Can you work these out from the model? Positions are in its coordinate system, mm. A direction names the side the tool comes from. Round coordinates to 2 decimals unless told otherwise and drop trailing zeros. Write each loop counter-clockwise with the first axis right and the second up, starting at its lowest first coordinate (ties: lowest second). Pieces come first, ordered by that corner, then holes. Notation, with made-up numbers: (83.5, 32.5) -> (101.5, 32.5) arc R17 cw to (101.5, 56.5) -> close; hole circle Ø11 at (6, -7). An arc over 180 degrees is marked (long way). Use CSV: the item, a comma, the result in double quotes.
```python
from build123d import *

# Parameters (mm, degrees)
SKETCH_1_W                   = 46
SKETCH_1_H                   = 26
EXTRUDE_1_DEPTH              = 5
SKETCH_2_W                   = 3
SKETCH_2_H                   = 26
EXTRUDE_2_DEPTH              = 34
FILLET_1_R                   = 13
CUT_EXTRUDE_1_REACH          = 63.693
SKETCH_3_R                   = 4
HOLE_WIZARD_M2_1_D           = 2.4
HOLE_WIZARD_M2_1_CBORE_D     = 4.4
HOLE_WIZARD_M2_1_CBORE_DEPTH = 2
SKETCH_6_W                   = 39
SKETCH_6_H                   = 25
CUT_EXTRUDE_3_DEPTH          = 3
CHAMFER_1_SIZE               = 3
SKETCH_7_W                   = 8
SKETCH_7_H                   = 5
CUT_EXTRUDE_4_DEPTH          = 10
SKETCH_8_W                   = 5
SKETCH_8_H                   = 5
CUT_EXTRUDE_5_DEPTH          = 10
SKETCH_9_R                   = 2.7
EXTRUDE_7_DEPTH              = 1
HOLE_WIZARD_M2_2_D           = 2.4
HOLE_WIZARD_M2_2_CBORE_D     = 4.4
HOLE_WIZARD_M2_2_CBORE_DEPTH = 2
M2X0_4_1_D                   = 1.6


with BuildPart() as part:
    # 草图1 → 凸台-拉伸1 (new body)
    with BuildSketch(Plane(origin=(0, 0, 0), x_dir=(1, 0, 0), z_dir=(0, 1, 0))):
        Rectangle(SKETCH_1_W, SKETCH_1_H)
    extrude(amount=EXTRUDE_1_DEPTH)

    # 草图2 → 凸台-拉伸2 (add)
    with BuildSketch(Plane(origin=(0, 5, 0), x_dir=(1, 0, 0), z_dir=(0, 1, 0))):
        with Locations((-21.5, 0)):
            Rectangle(SKETCH_2_W, SKETCH_2_H)
        with Locations((21.5, 0)):
            Rectangle(SKETCH_2_W, SKETCH_2_H)
    extrude(amount=EXTRUDE_2_DEPTH)

    # 圆角1
    fillet_1_edges = [part.edges().sort_by_distance(p)[0] for p in [
        (21.5, 39, -13),
        (-21.5, 39, -13),
        (21.5, 39, 13),
        (-21.5, 39, 13),
    ]]
    fillet(fillet_1_edges, radius=FILLET_1_R - 0.0001)  # a hair under: the kernel refuses the full size

    # 草图3 → 切除-拉伸1 (cut, up to next)
    with BuildSketch(Plane.ZY.offset(23), mode=Mode.PRIVATE) as cut_extrude_1_sk1:
        with Locations((0, 26)):
            Circle(SKETCH_3_R)
    cut_extrude_1_tool1 = extrude(cut_extrude_1_sk1.sketch, amount=-CUT_EXTRUDE_1_REACH, mode=Mode.PRIVATE) & part.part
    cut_extrude_1 = cut_extrude_1_tool1.solids().sort_by_distance((-23, 26, 0))[0]
    add(cut_extrude_1, mode=Mode.SUBTRACT)

    # M2 凹头盖螺钉的柱形沉头孔1 (through all)
    with Locations(Plane(origin=(-23, 26, -8), x_dir=(0, 0, -1), z_dir=(-1, 0, 0))):
        with Locations((0, 0), (-8, -8), (-16, 0), (-8, 8)):
            hole_wizard_m2_1 = CounterBoreHole(HOLE_WIZARD_M2_1_D / 2, HOLE_WIZARD_M2_1_CBORE_D / 2, HOLE_WIZARD_M2_1_CBORE_DEPTH)

    # 镜向1: 切除-拉伸1, M2 凹头盖螺钉的柱形沉头孔1 across plane
    add(cut_extrude_1.mirror(Plane(origin=(0, 0, 0), x_dir=(0, 0, 1), z_dir=(1, 0, 0))), mode=Mode.SUBTRACT)
    add(hole_wizard_m2_1.mirror(Plane(origin=(0, 0, 0), x_dir=(0, 0, 1), z_dir=(1, 0, 0))), mode=Mode.SUBTRACT)

    # 草图6 → 切除-拉伸3 (cut)
    with BuildSketch(Plane(origin=(0, 5, 0), x_dir=(1, 0, 0), z_dir=(0, 1, 0))):
        Rectangle(SKETCH_6_W, SKETCH_6_H)
    extrude(amount=-CUT_EXTRUDE_3_DEPTH, mode=Mode.SUBTRACT)

    # 倒角1
    chamfer_1_edges = [part.edges().sort_by_distance(p)[0] for p in [
        (-23, 0, 0),
        (23, 0, 0),
    ]]
    chamfer(chamfer_1_edges, length=CHAMFER_1_SIZE)

    # 草图7 → 切除-拉伸4 (cut)
    with BuildSketch(Plane(origin=(23, 0, 0), x_dir=(0, 0, -1), z_dir=(1, 0, 0))):
        with Locations((0, 3.5)):
            Rectangle(SKETCH_7_W, SKETCH_7_H)
    cut_extrude_4 = extrude(amount=-CUT_EXTRUDE_4_DEPTH, mode=Mode.SUBTRACT)

    # 镜向2: 切除-拉伸4 across plane
    add(cut_extrude_4.mirror(Plane(origin=(0, 0, 0), x_dir=(0, 0, 1), z_dir=(1, 0, 0))), mode=Mode.SUBTRACT)

    # 草图8 → 切除-拉伸5 (cut)
    with BuildSketch(Plane(origin=(0, 2, 0), x_dir=(1, 0, 0), z_dir=(0, 1, 0))):
        Rectangle(SKETCH_8_W, SKETCH_8_H)
    extrude(amount=-CUT_EXTRUDE_5_DEPTH, mode=Mode.SUBTRACT)

    # 草图9 → 凸台-拉伸7 (add)
    with BuildSketch(Plane(origin=(0, 2, 0), x_dir=(1, 0, 0), z_dir=(0, 1, 0))):
        with Locations(Location((-5, 5, 0), (0, 0, 270))):
            Circle(SKETCH_9_R)
        with Locations(Location((5, 5, 0), (0, 0, 270))):
            Circle(SKETCH_9_R)
        with Locations(Location((5, -5, 0), (0, 0, 270))):
            Circle(SKETCH_9_R)
        with Locations(Location((-5, -5, 0), (0, 0, 270))):
            Circle(SKETCH_9_R)
    extrude(amount=EXTRUDE_7_DEPTH)

    # M2 凹头盖螺钉的柱形沉头孔2 (through all)
    with Locations(Plane(origin=(-5, 3, 5), x_dir=(0, 0, 1), z_dir=(0, 1, 0))):
        with Locations((0, 0), (0, 10), (-10, 10), (-10, 0)):
            CounterBoreHole(HOLE_WIZARD_M2_2_D / 2, HOLE_WIZARD_M2_2_CBORE_D / 2, HOLE_WIZARD_M2_2_CBORE_DEPTH)

    # M2x0.4 螺纹孔1 (through all)
    with Locations(Plane(origin=(-5, 2, 0), x_dir=(0, 0, 1), z_dir=(0, 1, 0))):
        with Locations((0, 0), (-5, 5), (0, 10), (5, 5)):
            Hole(M2X0_4_1_D / 2)


solid = part.part
```
Q1. Please list where these lines run through material, in increasing order: probe 1 along Y at (x, z) = (22.1, 0); probe 2 along X at (y, z) = (20.5, -5.25); probe 3 along Z at (x, y) = (22.2, 18).
Resolved:
probe 1,"y = 6 to 15.8, 20.2 to 22, 30 to 31.8, 36.2 to 39"
probe 2,"x = -23 to -20, 20 to 23"
probe 3,"z = -13 to -2.2, 2.2 to 13"
Q2. On a 3-axis mill with a long thin cutter (end or side, diameter ignored), from which of +Z, -Z, +X, -X, +Y, -Y can I reach the whole of each face in a straight line? I mean faces 1 (the face through (-2.5, 1, 0)), 2 (the face through (-20.49, 32.81, -0.16)), 3 (the face through (-21, 27, -9)), 4 (the face through (4, 1, -4)), 5 (the face through (20, 3, -4)). Say none if no direction works.
Resolved:
face 1,"+Y, -Y"
face 2,"+X, -X"
face 3,"-X"
face 4,"+Y"
face 5,"+X"
Q3. Suppose I cut it at C-C (y = 18). Write out the boundary of the cut face in (x, z).
Resolved:
outline,"(-23, -13) -> (-20, -13) -> (-20, -1.2) -> (-21, -1.2) -> (-21, -2.2) -> (-23, -2.2) -> close; (-23, 2.2) -> (-21, 2.2) -> (-21, 1.2) -> (-20, 1.2) -> (-20, 13) -> (-23, 13) -> close; (20, -13) -> (23, -13) -> (23, -2.2) -> (21, -2.2) -> (21, -1.2) -> (20, -1.2) -> close; (20, 1.2) -> (21, 1.2) -> (21, 2.2) -> (23, 2.2) -> (23, 13) -> (20, 13) -> close"
Q4. Will these pins go through, and if not, where does the flat tip stop? P1, Ø2, axis at x = 5, z = 6, coming from the +Y side; P2, Ø3, axis at x = -12.5, z = 9.5, coming from the +Y side; P3, Ø5, axis at x = 6, z = -5.5, coming from the +Y side.
Resolved:
P1,"stops at y = 1"
P2,"stops at y = 2"
P3,"stops at y = 3"
Q5. Suppose I cut it at B-B (x = 0). Write out the boundary of the cut face in (y, z), and give its area (3 significant figures).
Resolved:
outline,"(0, -13) -> (5, -13) -> (5, -12.5) -> (2, -12.5) -> (2, -5.8) -> (0, -5.8) -> close; (0, -4.2) -> (2, -4.2) -> (2, -2.5) -> (0, -2.5) -> close; (0, 2.5) -> (2, 2.5) -> (2, 4.2) -> (0, 4.2) -> close; (0, 5.8) -> (2, 5.8) -> (2, 12.5) -> (5, 12.5) -> (5, 13) -> (0, 13) -> close"
area,"38.6 mm^2"
Q6. If we mould it in two halves opening along Z, with no side actions, what happens to faces 6 (the face through (17, 1, 0)), 7 (the face through (-4.95, 0.49, -3.8)), 8 (the face through (-0.09, 5, -12.85))? For each: released by +Z, released by -Z, zero draft, split by the parting line, or undercut.
Resolved:
face 6,"undercut"
face 7,"undercut"
face 8,"zero draft"
Q7. Suppose I cut it at D-D (x = -18.5). Write out the boundary of the cut face in (y, z), and give its area (3 significant figures).
Resolved:
outline,"(0, -13) -> (5, -13) -> (5, -12.5) -> (2, -12.5) -> (2, -4) -> (1, -4) -> (1, 4) -> (2, 4) -> (2, 12.5) -> (5, 12.5) -> (5, 13) -> (0, 13) -> close"
area,"47.0 mm^2"
Q8. Suppose I cut it at A-A (y = 9.5). Write out the boundary of the cut face in (x, z), and give its area (3 significant figures).
Resolved:
outline,"(-23, -13) -> (-20, -13) -> (-20, 13) -> (-23, 13) -> close; (20, -13) -> (23, -13) -> (23, 13) -> (20, 13) -> close"
area,"156 mm^2"
